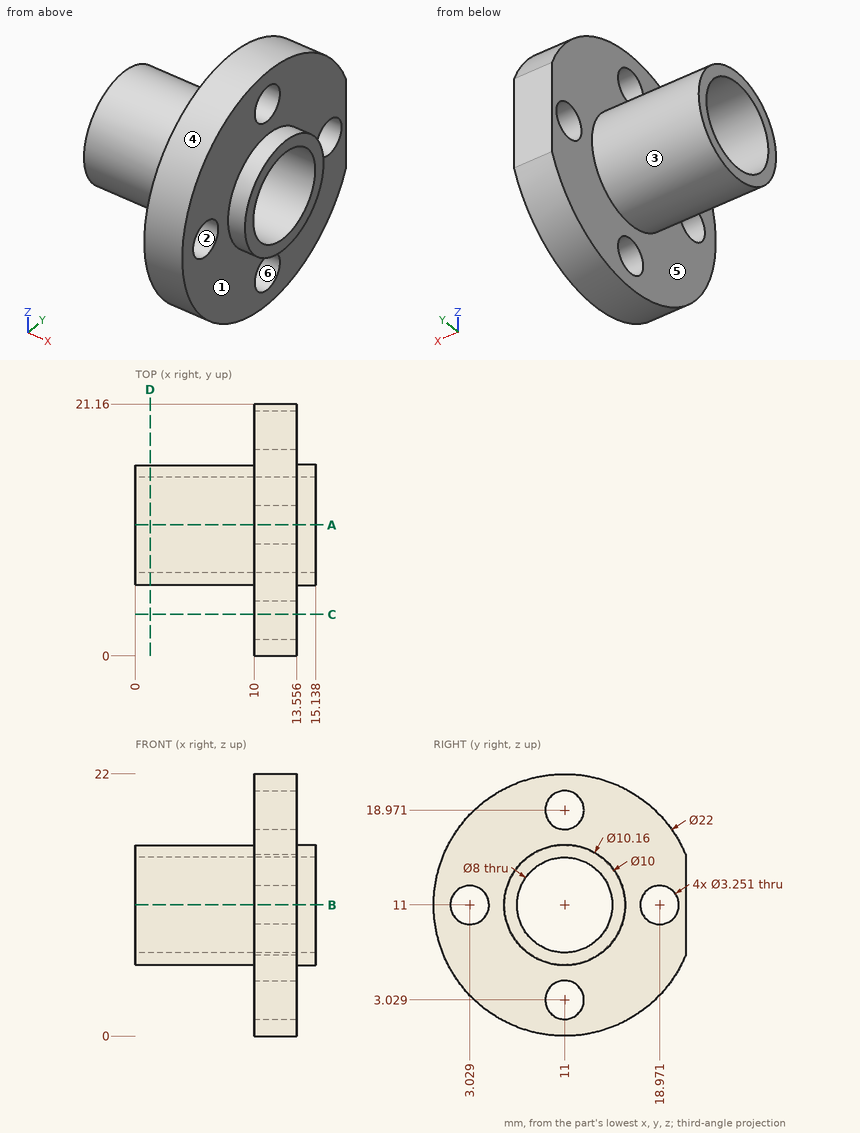
Here's the drawing with two shaded views (mm, measured from the low corner). I have some questions. A direction names the side the tool comes from. Coordinates: 2 decimals unless noted, no trailing zeros. Order: outer loops, then holes, each group sorted by start corner. A loop starts at its lowest first (then second) coordinate and runs counter-clockwise, first axis right, second up.
Q1. Thinking about a two-plate mould opening in Z: for the marked faces 4, 5 and 6, which applies, released by +Z, released by -Z, zero draft, split by the parting line, or undercut?
Q2. Suppose I cut it at C-C on y = 3.5. Please give me the cut outline in (x, z).
Q3. Suppose I cut it at B-B on z = 11. Please give me the cut outline in (x, y) (1 decimal).
Q4. Suppose I cut it at A-A on y = 11. Please give me the cut outline in (x, z) (1 decimal).
Q5. Will these pins go through, and if not, where does the flat tip stop? pin 1 (1 mm diameter, centred on y = 7, z = 3, fed in from +X); pin 2 (2 mm diameter, centred on x = 10.5, y = 14, fed in from +Z); pin 3 (4 mm diameter, centred on x = 5, y = 16.5, fed in from -Z).
Q6. Please list where these lines run through material, in increasing order: L1, parallel to Z at x = 12.7, y = 11 (1 decimal); L2, parallel to Z at x = 5.5, y = 11.
Q7. Suppose I cut it at D-D on x = 1.25. Please give me the cut outline in (y, z).
Q8. Which directions (+Z, -Z, +X, -X, +Y, -Y) give clear straight access to the entire face, cutting with the end or side of a thin tool? Please do the marked faces 1, 2 and 3.
Answer:
1. face 4: split by the parting line
1. face 5: zero draft
1. face 6: undercut
2. outline: (10, 2.95) - (13.56, 2.95) - (13.56, 9.44) - (10, 9.44) - close; (10, 12.56) - (13.56, 12.56) - (13.56, 19.05) - (10, 19.05) - close
3. outline: (0, 6) - (10, 6) - (10, 4.7) - (13.6, 4.7) - (13.6, 5.9) - (15.1, 5.9) - (15.1, 7) - (0, 7) - close; (0, 15) - (15.1, 15) - (15.1, 16.1) - (13.6, 16.1) - (13.6, 17.3) - (10, 17.3) - (10, 16) - (0, 16) - close; (10, 0) - (13.6, 0) - (13.6, 1.4) - (10, 1.4) - close; (10, 20.6) - (13.6, 20.6) - (13.6, 21.2) - (10, 21.2) - close
4. outline: (0, 6) - (10, 6) - (10, 4.7) - (13.6, 4.7) - (13.6, 5.9) - (15.1, 5.9) - (15.1, 7) - (0, 7) - close; (0, 15) - (15.1, 15) - (15.1, 16.1) - (13.6, 16.1) - (13.6, 17.3) - (10, 17.3) - (10, 16) - (0, 16) - close; (10, 0) - (13.6, 0) - (13.6, 1.4) - (10, 1.4) - close; (10, 20.6) - (13.6, 20.6) - (13.6, 22) - (10, 22) - close
5. pin 1: stops at x = 13.56
5. pin 2: stops at z = 21.82
5. pin 3: stops at z = 7.43
6. L1: z = 0 to 1.4, 4.7 to 7, 15 to 17.3, 20.6 to 22
6. L2: z = 6 to 7, 15 to 16
7. outline: circle Ø10 at (11, 11); hole circle Ø8 at (11, 11)
8. face 1: +X
8. face 2: +X, -X
8. face 3: -X
